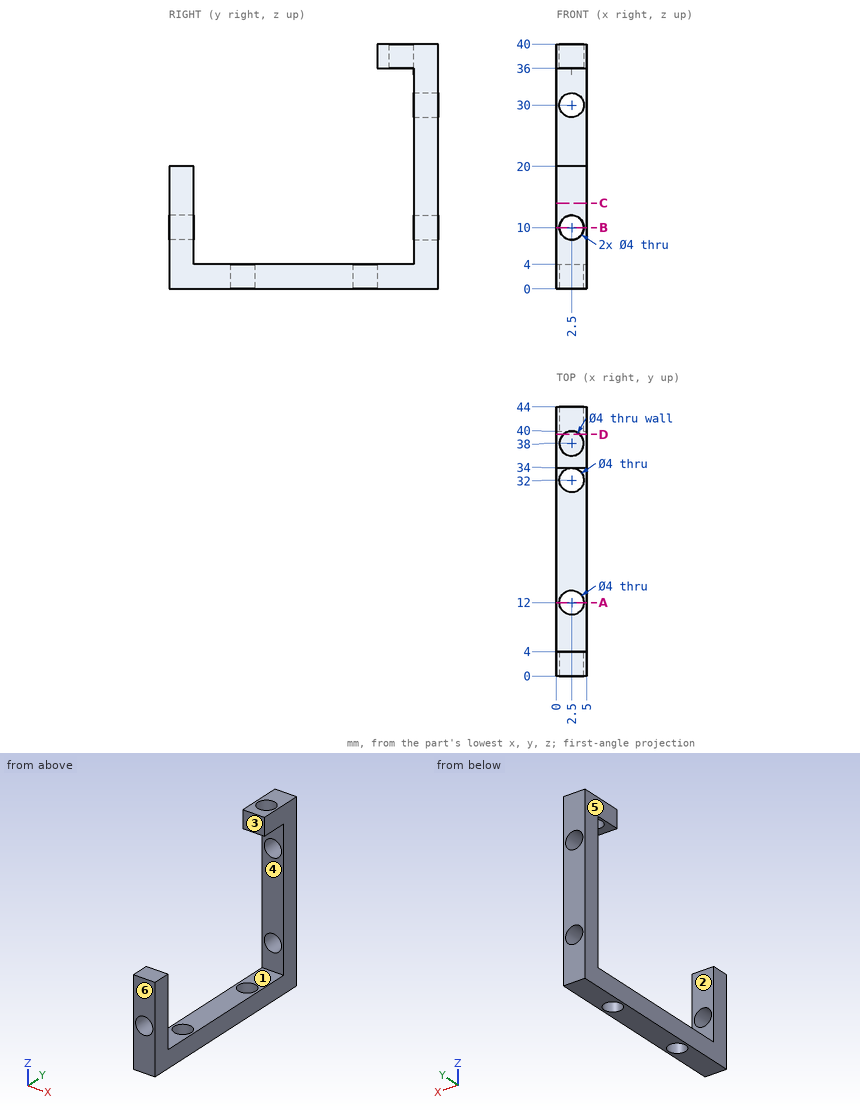
Geometry: see drawing. Coordinates: mm, zero at the bounding-box minimum. A direction names the side the tool comes from. Give positions to 0.01 mm unless a question says otherwise; leave off trailing zeros. Write each loop counter-clockwise with the first axis right and the second up, starting at its lowest first coordinate (ties: lowest second). Pieces come first, ordered by that corner, then holes. Notation, with made-up numbers: (86.5, 8) -> (100.5, 8) arc R33 ccw to (100.5, 46) -> close; hole circle Ø5 at (-33, -30). An arc over 180 degrees is marked (long way). Use one line per item in the form item = value. Start each with the question number.
1) Ray query, probe 1 along Z at (x, y) = (2.5, 42.1); probe 2 along X at (y, z) = (38, 37); probe 3 along Y at (x, z) = (4.4, 12). Return the intervals inside material, ascending. Write a range as from..to.
2) Pin query (flat end, axial travel): pin 1 (2 mm diameter, centred on x = 2.5, y = 1.5, fed in from +Z); pin 2 (1 mm diameter, centred on x = 2.5, y = 27, fed in from +Z). Return the tip coordinate at first contact, or that it passes through.
3) Section query B-B on z = 10. Return the cut outline in (x, y), then the cut area to 3 significant figures.
4) Section query D-D on y = 39.5. Return the cut outline in (x, z), then the cut area to 3 significant figures.
5) Section query C-C on z = 14. Return the cut outline in (x, y).
6) Section query A-A on y = 12. Return the cut outline in (x, z).
7) Set-up query: the marked faces 1, 2 and 3. Return all of +Z, -Z, +X, -X, +Y, -Y with unobstructed straight access to the full face (end or side cutting, diameter ignored); none if empty.
8) Draft query along Y for the marked faces 4, 5 and 6. Return one class per face: pulls with the +Y half, pulls with the -Y half, needs draft (parallel to the pull), parting line crosses it, or undercut.
Outcome:
q1.probe_1 = 0..8, 12..28, 32..40
q1.probe_2 = 0..0.5, 4.5..5
q1.probe_3 = 0..4, 40..44
q2.pin_1 = 20
q2.pin_2 = 4
q3.outline = (0, 0) -> (0.5, 0) -> (0.5, 4) -> (0, 4) -> close; (0, 40) -> (0.5, 40) -> (0.5, 44) -> (0, 44) -> close; (4.5, 0) -> (5, 0) -> (5, 4) -> (4.5, 4) -> close; (4.5, 40) -> (5, 40) -> (5, 44) -> (4.5, 44) -> close
q3.area = 8.00 mm^2
q4.outline = (0, 0) -> (5, 0) -> (5, 4) -> (0, 4) -> close; (0, 36) -> (1.18, 36) -> (1.18, 40) -> (0, 40) -> close; (3.82, 36) -> (5, 36) -> (5, 40) -> (3.82, 40) -> close
q4.area = 29.4 mm^2
q5.outline = (0, 0) -> (5, 0) -> (5, 4) -> (0, 4) -> close; (0, 40) -> (5, 40) -> (5, 44) -> (0, 44) -> close
q6.outline = (0, 0) -> (0.5, 0) -> (0.5, 4) -> (0, 4) -> close; (4.5, 0) -> (5, 0) -> (5, 4) -> (4.5, 4) -> close
q7.face_1 = +X, -X
q7.face_2 = +Z, +X, -X
q7.face_3 = +Z, +X, -X, -Y
q8.face_4 = undercut
q8.face_5 = needs draft
q8.face_6 = pulls with the -Y half
